from build123d import *

# Parameters (mm, degrees)
SCHIZZO1_R                                           = 109.75
SCHIZZO1_R_2                                         = 7.5
ESTRUSIONE_ESTRUSIONE1_DEPTH                         = 180
FORO_LAMATO_PER_BULLONE_M5_A_TESTA_ESAGO_D           = 5.4
FORO_LAMATO_PER_BULLONE_M5_A_TESTA_ESAGO_DEPTH       = 20
FORO_LAMATO_PER_BULLONE_M5_A_TESTA_ESAGO_CBORE_D     = 10
FORO_LAMATO_PER_BULLONE_M5_A_TESTA_ESAGO_CBORE_DEPTH = 3
FORO_LAMATO_PER_BULLONE_M5_A_TESTA_ESAGO_TIP         = 1.622323671
FORO_LAMATO_PER_BULLONE_M5_A_TESTA_E_2_D             = 5.4
FORO_LAMATO_PER_BULLONE_M5_A_TESTA_E_2_DEPTH         = 20
FORO_LAMATO_PER_BULLONE_M5_A_TESTA_E_2_CBORE_D       = 10
FORO_LAMATO_PER_BULLONE_M5_A_TESTA_E_2_CBORE_DEPTH   = 3
FORO_LAMATO_PER_BULLONE_M5_A_TESTA_E_2_TIP           = 1.622323671
FORO_LAMATO_PER_BULLONE_M5_A_TESTA_E_3_D             = 5.4
FORO_LAMATO_PER_BULLONE_M5_A_TESTA_E_3_DEPTH         = 20
FORO_LAMATO_PER_BULLONE_M5_A_TESTA_E_3_CBORE_D       = 10
FORO_LAMATO_PER_BULLONE_M5_A_TESTA_E_3_CBORE_DEPTH   = 3
FORO_LAMATO_PER_BULLONE_M5_A_TESTA_E_3_TIP           = 1.622323671
FORO_LAMATO_PER_BULLONE_M5_A_TESTA_E_4_D             = 5.4
FORO_LAMATO_PER_BULLONE_M5_A_TESTA_E_4_DEPTH         = 20
FORO_LAMATO_PER_BULLONE_M5_A_TESTA_E_4_CBORE_D       = 10
FORO_LAMATO_PER_BULLONE_M5_A_TESTA_E_4_CBORE_DEPTH   = 3
FORO_LAMATO_PER_BULLONE_M5_A_TESTA_E_4_TIP           = 1.622323671
ESTRUSIONE_ESTRUSIONE2_DEPTH                         = 20
ESTRUSIONE_ESTRUSIONE3_DEPTH                         = 10
SMUSSO1_SIZE                                         = 10
RACCORDO1_R                                          = 10
SMUSSO2_SIZE                                         = 2


with BuildPart() as part:
    # Schizzo1 → Estrusione-Estrusione1 (new body)
    with BuildSketch(Plane(origin=(0, 0, 0), x_dir=(1, 0, 0), z_dir=(0, 1, 0))):
        with Locations(Location((0, 0, 0), (0, 0, 90))):
            Circle(SCHIZZO1_R)
        with Locations(Location((0, 98, 0), (0, 0, 90))):
            Circle(SCHIZZO1_R_2, mode=Mode.SUBTRACT)
        with BuildLine():
            Line((-16.652598983, 96.067377122), (-5, 89.339745962))
            ThreePointArc((-5, 89.339745962), (0, 88), (5, 89.339745962))
            Line((5, 89.339745962), (16.652598983, 96.067377122))
            ThreePointArc((16.652598983, 96.067377122), (0, -97.5), (-16.652598983, 96.067377122))
        make_face(mode=Mode.SUBTRACT)
    extrude(amount=ESTRUSIONE_ESTRUSIONE1_DEPTH)

    # Foro lamato per Bullone M5 a testa esagonale-1
    with Locations(Plane(origin=(-77.604969235, 170, -77.604969235), x_dir=(-0.707106781187, 0, 0.707106781187), z_dir=(-0.707106781187, 0, -0.707106781187))):
        with Locations((0, 0)):
            CounterBoreHole(FORO_LAMATO_PER_BULLONE_M5_A_TESTA_ESAGO_D / 2, FORO_LAMATO_PER_BULLONE_M5_A_TESTA_ESAGO_CBORE_D / 2, FORO_LAMATO_PER_BULLONE_M5_A_TESTA_ESAGO_CBORE_DEPTH, depth=FORO_LAMATO_PER_BULLONE_M5_A_TESTA_ESAGO_DEPTH)
            with Locations((0, 0, -(FORO_LAMATO_PER_BULLONE_M5_A_TESTA_ESAGO_DEPTH + FORO_LAMATO_PER_BULLONE_M5_A_TESTA_ESAGO_TIP / 2))):  # 118° drill point
                Cone(0, FORO_LAMATO_PER_BULLONE_M5_A_TESTA_ESAGO_D / 2, FORO_LAMATO_PER_BULLONE_M5_A_TESTA_ESAGO_TIP, mode=Mode.SUBTRACT)

    # Foro lamato per Bullone M5 a testa e 2
    with Locations(Plane(origin=(-77.604969235, 170, 77.604969235), x_dir=(0.707106781187, 0, 0.707106781187), z_dir=(-0.707106781187, 0, 0.707106781187))):
        with Locations((0, 0)):
            CounterBoreHole(FORO_LAMATO_PER_BULLONE_M5_A_TESTA_E_2_D / 2, FORO_LAMATO_PER_BULLONE_M5_A_TESTA_E_2_CBORE_D / 2, FORO_LAMATO_PER_BULLONE_M5_A_TESTA_E_2_CBORE_DEPTH, depth=FORO_LAMATO_PER_BULLONE_M5_A_TESTA_E_2_DEPTH)
            with Locations((0, 0, -(FORO_LAMATO_PER_BULLONE_M5_A_TESTA_E_2_DEPTH + FORO_LAMATO_PER_BULLONE_M5_A_TESTA_E_2_TIP / 2))):  # 118° drill point
                Cone(0, FORO_LAMATO_PER_BULLONE_M5_A_TESTA_E_2_D / 2, FORO_LAMATO_PER_BULLONE_M5_A_TESTA_E_2_TIP, mode=Mode.SUBTRACT)

    # Foro lamato per Bullone M5 a testa e 3
    with Locations(Plane(origin=(77.604969235, 170, -77.604969235), x_dir=(-0.707106781187, 0, -0.707106781187), z_dir=(0.707106781187, 0, -0.707106781187))):
        with Locations((0, 0)):
            CounterBoreHole(FORO_LAMATO_PER_BULLONE_M5_A_TESTA_E_3_D / 2, FORO_LAMATO_PER_BULLONE_M5_A_TESTA_E_3_CBORE_D / 2, FORO_LAMATO_PER_BULLONE_M5_A_TESTA_E_3_CBORE_DEPTH, depth=FORO_LAMATO_PER_BULLONE_M5_A_TESTA_E_3_DEPTH)
            with Locations((0, 0, -(FORO_LAMATO_PER_BULLONE_M5_A_TESTA_E_3_DEPTH + FORO_LAMATO_PER_BULLONE_M5_A_TESTA_E_3_TIP / 2))):  # 118° drill point
                Cone(0, FORO_LAMATO_PER_BULLONE_M5_A_TESTA_E_3_D / 2, FORO_LAMATO_PER_BULLONE_M5_A_TESTA_E_3_TIP, mode=Mode.SUBTRACT)

    # Foro lamato per Bullone M5 a testa e 4
    with Locations(Plane(origin=(77.604969235, 170, 77.604969235), x_dir=(0.707106781187, 0, -0.707106781187), z_dir=(0.707106781187, 0, 0.707106781187))):
        with Locations((0, 0)):
            CounterBoreHole(FORO_LAMATO_PER_BULLONE_M5_A_TESTA_E_4_D / 2, FORO_LAMATO_PER_BULLONE_M5_A_TESTA_E_4_CBORE_D / 2, FORO_LAMATO_PER_BULLONE_M5_A_TESTA_E_4_CBORE_DEPTH, depth=FORO_LAMATO_PER_BULLONE_M5_A_TESTA_E_4_DEPTH)
            with Locations((0, 0, -(FORO_LAMATO_PER_BULLONE_M5_A_TESTA_E_4_DEPTH + FORO_LAMATO_PER_BULLONE_M5_A_TESTA_E_4_TIP / 2))):  # 118° drill point
                Cone(0, FORO_LAMATO_PER_BULLONE_M5_A_TESTA_E_4_D / 2, FORO_LAMATO_PER_BULLONE_M5_A_TESTA_E_4_TIP, mode=Mode.SUBTRACT)



with BuildPart() as body_2:
    # Schizzo1<4> → Estrusione-Estrusione2 (new body)
    with BuildSketch(Plane(origin=(0, 0, 0), x_dir=(1, 0, 0), z_dir=(0, 1, 0))):
        with BuildLine():
            Line((-25, 85.937477273), (-21.68001113, 95.059071726))
            ThreePointArc((-21.68001113, 95.059071726), (0, -97.5), (21.68001113, 95.059071726))
            Line((21.68001113, 95.059071726), (25, 85.937477273))
            ThreePointArc((25, 85.937477273), (0, -89.5), (-25, 85.937477273))
        make_face()
    extrude(amount=-ESTRUSIONE_ESTRUSIONE2_DEPTH)


with BuildPart() as part_1:
    add(part.part)

    add(body_2.part)  # Estrusione-Estrusione3 merges body 2
    # Schizzo1<5> → Estrusione-Estrusione3 (add)
    with BuildSketch(Plane(origin=(0, 0, 0), x_dir=(1, 0, 0), z_dir=(0, 1, 0))):
        with BuildLine():
            Line((-25, 85.937477273), (-21.68001113, 95.059071726))
            ThreePointArc((-21.68001113, 95.059071726), (0, -97.5), (21.68001113, 95.059071726))
            Line((21.68001113, 95.059071726), (25, 85.937477273))
            ThreePointArc((25, 85.937477273), (0, -89.5), (-25, 85.937477273))
        make_face()
    extrude(amount=ESTRUSIONE_ESTRUSIONE3_DEPTH)

    # Smusso1
    # the kernel refuses this chamfer: 10 mm, written as the material it takes off along each edge
    with BuildSketch(Plane(origin=(0, 10, 0), x_dir=(0.0031415874858797023, 0, -0.9999950652018582), z_dir=(-0.9999950652018582, 0, -0.0031415874858797023))) as smusso1_piece_1_section:
        Polygon((89.5, SMUSSO1_SIZE), (89.5 + SMUSSO1_SIZE, 0), (89.5, 0), align=None)
    smusso1_piece_1 = revolve(axis=Axis((0, 10, 0), (0, -1, 0)), revolution_arc=359.64, mode=Mode.PRIVATE)
    smusso1_piece_1 = smusso1_piece_1 & Plane(origin=(0, 6.636633225, 0), x_dir=(0.17079588700932372, 0, -0.9853064320203632), z_dir=(0, -1, 0)) * Cylinder(97.5, 399, mode=Mode.PRIVATE)
    smusso1_piece_1 = split(smusso1_piece_1, bisect_by=Plane(origin=(35.757086514, 6.636633225, -107.09735814), z_dir=(0.5000000000000053, 0, 0.8660254037844358)), keep=Keep.TOP, mode=Mode.PRIVATE)
    add(smusso1_piece_1, mode=Mode.SUBTRACT)
    with BuildSketch(Plane(origin=(0, 10, 0), x_dir=(0.0031415874858797023, 0, -0.9999950652018582), z_dir=(-0.9999950652018582, 0, -0.0031415874858797023))) as smusso1_piece_2_section:
        Polygon((89.5, SMUSSO1_SIZE), (89.5 + SMUSSO1_SIZE, 0), (89.5, 0), align=None)
    smusso1_piece_2 = revolve(axis=Axis((0, 10, 0), (0, -1, 0)), revolution_arc=359.64, mode=Mode.PRIVATE)
    smusso1_piece_2 = smusso1_piece_2 & Plane(origin=(0, 6.636633226, 0), x_dir=(0.17079588700932372, 0, -0.9853064320203632), z_dir=(0, -1, 0)) * Cylinder(97.5, 399, mode=Mode.PRIVATE)
    smusso1_piece_2 = split(smusso1_piece_2, bisect_by=Plane(origin=(-34.569971333, 6.636633226, -59.64419713), z_dir=(-0.9396926207859074, 0, -0.3420201433256714)), keep=Keep.TOP, mode=Mode.PRIVATE)
    add(smusso1_piece_2, mode=Mode.SUBTRACT)

    # Raccordo1
    raccordo1_edges = [part_1.edges().sort_by_distance(p)[0] for p in [
        (-16.652598983, 90, -96.067377122),
        (16.652598983, 90, -96.067377122),
    ]]
    fillet(raccordo1_edges, radius=RACCORDO1_R)

    # Smusso2
    smusso2_edges = [part_1.edges().sort_by_distance(p)[0] for p in [
        (0, -20, 97.5),
        (0, -20, 89.5),
    ]]
    chamfer(smusso2_edges, length=SMUSSO2_SIZE)


solid = part_1.part
For this review, take the finished solid that the model builds, in its own axes (mm). A direction names the side the tool comes from. Round coordinates to 2 decimals unless told otherwise and drop trailing zeros. Write each loop counter-clockwise with the first axis right and the second up, starting at its lowest first coordinate (ties: lowest second). Pieces come first, ordered by that corner, then holes. Notation, with made-up numbers: (-16.75, -13.5) -> (35.25, -13.5) arc R34 ccw to (35.25, 22.5) -> close; hole circle Ø8 at (62.5, -3). An arc over 180 degrees is marked (long way). Put each result on its own line as item: value.
Q1. The part is to be moulded in two halves that separate along Z. For faces 1 (the cylindrical face through (-3.98, -8.87, 97.42)), 2 (the cylindrical face through (-77.019, 174.957, 76.099)), 3 (the flat face through (-1, 0, -89)), say which applies: released by +Z, released by -Z, zero draft, split by the parting line, or undercut.
Determined:
face 1: split by the parting line
face 2: undercut
face 3: zero draft
Q2. Consider section A-A on x = 0. State the section outline as (y, z) points, and give its area (3 significant figures).
Determined:
outline: (-20, 91.5) -> (-18, 89.5) -> (0, 89.5) -> (8, 97.5) -> (180, 97.5) -> (180, 109.75) -> (0, 109.75) -> (0, 97.5) -> (-18, 97.5) -> (-20, 95.5) -> close; (0, -109.75) -> (180, -109.75) -> (180, -105.5) -> (0, -105.5) -> close; (0, -90.5) -> (180, -90.5) -> (180, -88) -> (0, -88) -> close
area: 3,610 mm^2
Q3. Clearance check with flat-ended pins moving along their axes: pin 1 Ø1 at (x, y) = (-32.5, 29) entering from -Z; pin 2 Ø1.5 at (x, y) = (84, 45) entering from +Z; pin 3 Ø6 at (x, z) = (72, -60) entering from +Y. State where each tip first meets the part, or that it passes through.
Determined:
pin 1: stops at z = -104.98
pin 2: stops at z = 71.52
pin 3: stops at y = 7.22
Q4. Consider section C-C on y = 143. State the section outline as (x, z) points.
Determined:
outline: circle Ø219.5 at (0, 0); hole (-20.52, -95.32) arc R10 ccw to (-13.42, -94.2) -> (-5, -89.34) arc R10 cw to (5, -89.34) -> (13.42, -94.2) arc R10 ccw to (20.52, -95.32) arc R97.5 ccw (long way) to start; hole circle Ø15 at (0, -98)
Q5. Machinability: for faces 4 (the flat face through (-1, 180, -89)), 5 (the flat face through (-77.01, 167.85, -73.96)), 6 (the flat face through (-9.268, 88.74, -91.804)), which of the approach directions +Z, -Z, +X, -X, +Y, -Y give a long, thin tool a straight path to every point of the face, cutting with its end or side? Answer none if there is none.
Determined:
face 4: +Z, -Z, +X, -X, +Y
face 5: none
face 6: +Y, -Y
Q6. Consider section B-B on z = 0. State the section outline as (x, y) points, and give its area (3 significant figures).
Determined:
outline: (-109.75, 0) -> (-97.5, 0) -> (-97.5, -18) -> (-95.5, -20) -> (-91.5, -20) -> (-89.5, -18) -> (-89.5, 0) -> (-97.5, 8) -> (-97.5, 180) -> (-109.75, 180) -> close; (89.5, -18) -> (91.5, -20) -> (95.5, -20) -> (97.5, -18) -> (97.5, 0) -> (109.75, 0) -> (109.75, 180) -> (97.5, 180) -> (97.5, 8) -> (89.5, 0) -> close
area: 4,790 mm^2
Q7. To check wall thickness, follow L1, parallel to Z at x = -2, y = 80; L2, parallel to X at y = -5, z = 0; L3, parallel to Y at x = -93, z = 48.5. State the ranges of each line that lie inside material, in increasing order. Write a range as [from, to].
Determined:
L1: z = [-109.73, -105.23], [-90.77, -88.2], [97.48, 109.73]
L2: x = [-97.5, -89.5], [89.5, 97.5]
L3: y = [0, 180]
